Autodesk Inventor part; units mm, degrees
ref_plane "MSC_PT1" through (0, 0, 1.8) normal (0, 0, 1) x (1, 0, 0)
ref_plane "MSC_PT2" through (0, 0, 0) normal (0, 0, -1) x (-1, 0, 0)
ref_plane "MSC_PF1" through (0, 0, 0) normal (1, 0, 0) x (0, 1, 0)
sketch "Sketch1" plane through (0, 0, 0) normal (0, 0, 1) x (1, 0, 0)
  circle A0 centre (0, 0) radius 2.75 construction
  line L0 (-2.75, 1.5877) -> (-2.75, -1.5877)
  line L1 (-2.75, -1.5877) -> (0, -3.1754)
  line L2 (0, -3.1754) -> (2.75, -1.5877)
  line L3 (2.75, -1.5877) -> (2.75, 1.5877)
  line L4 (2.75, 1.5877) -> (0, 3.1754)
  line L5 (0, 3.1754) -> (-2.75, 1.5877)
  line L6 (0, 4.4456) -> (0, -4.4456)
  line L7 (-3.85, 0) -> (3.85, 0)
  point P0 (0, 0)
  dimension "ParS" = 5.5
extrude "Extrusion1" add sketch "Sketch1" along normal blind 1.8
sketch "Sketch2" plane through (0, 0, 1.8) normal (0, 0, 1) x (1, 0, 0)
  point P0 (0, 0)
  point P1 (0, 0)
hole "Hole1" at (0, 0, 1.8) direction (0, 0, -1) diameter 2.459 end through all
ref_plane "MSC_PT1" through (0, 0, 1.8) normal (0, 0, 1) x (1, 0, 0)
ref_plane "MSC_PT2" through (0, 0, 0) normal (0, 0, -1) x (-1, 0, 0)
ref_plane "MSC_PF1" through (0, 0, 0) normal (1, 0, 0) x (0, 1, 0)
chamfer "Chamfer1" distance 0.3 angle 45 2 edges at (0, 1.2295, 1.8) (0, 1.2295, 0)
equation "\"d17\" = 0.6 * PTC"
equation "\"d18\" = 0.6 * PTC"
equation "\"d4\" = M"
equation "\"PTC\" = 0.5"
equation "\"NND\" = 3"
equation "\"THREADDIA\" = NND"
properties part number "ISO 4036 - M3" material "Steel, Mild"
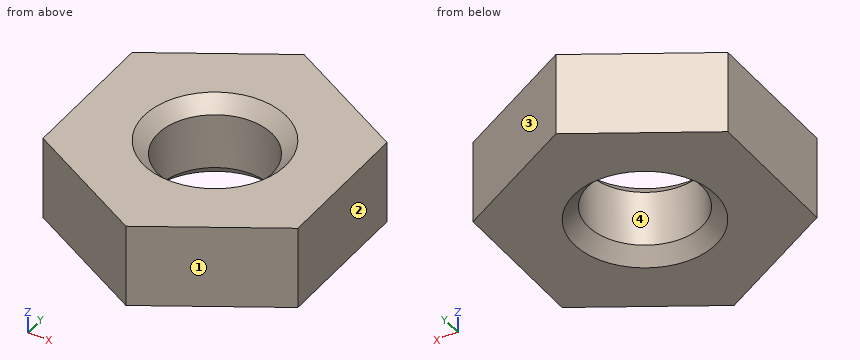
The listing builds one solid part. Answer for the finished solid, in the listing's coordinates (mm). Face numbers are marked on the shaded views. Round coordinates to 2 decimals unless told otherwise and drop trailing zeros. Loops run counter-clockwise (first coordinate to the right, second up) from the corner with the lowest first, then second, coordinate; pieces in that order, holes last. Notation, with made-up numbers: M 20.25,38 L 39.25,38 A12 ccw 39.25,61 Z; hole C 38,38.5 d1. An arc over 180 degrees is marked long. Write each question's results on one line, items separated by ' | '. Start each with the question number.
1) Find section D-D on y = -2. Write down the section's boundary in (x, z), plus the area to 3 significant figures.
2) Determine the mould class of the marked faces 1, 2, 3 and 4 for opening direction Y: pulls with the +Y half, pulls with the -Y half, needs draft (parallel to the pull), parting line crosses it, or undercut.
3) Find section C-C on z = 0.2. Write down the section's boundary in (x, y), plus the area to 3 significant figures.
4) Straight lines are drawn through the part: probe 1 along X at (y, z) = (0, 0.7); probe 2 along Y at (x, z) = (0.9, 1.05); probe 3 along X at (y, z) = (-0.5, 1.15). For each, find the intervals that lie inside material, in ascending order.
5) Find section B-B on y = 0. Write down the section's boundary in (x, z).
6) Each of these flat-tipped pins is pushed along its axis until it touches: pin 1 (1 mm diameter, centred on x = 1, z = 1, fed in from -Y); pin 2 (3 mm diameter, centred on x = 0, y = 0, fed in from +Z); pin 3 (1 mm diameter, centred on x = 1.5, z = 0.5, fed in from -Y). Where does it stop, or does it pass through?
7) Find section A-A on z = 0.75. Write down the section's boundary in (x, y), plus the area to 3 significant figures.
Final values:
1) outline: M -2.04,0 L 2.04,0 L 2.04,1.8 L -2.04,1.8 Z | area: 7.33 mm²
2) face 1: pulls with the -Y half | face 2: needs draft | face 3: pulls with the +Y half | face 4: undercut
3) outline: M -2.75,-1.59 L 0,-3.18 L 2.75,-1.59 L 2.75,1.59 L 0,3.18 L -2.75,1.59 Z; hole C 0,0 d2.66 | area: 20.6 mm²
4) probe 1: -2.75 to -1.23, 1.23 to 2.75 | probe 2: -2.66 to -0.84, 0.84 to 2.66 | probe 3: -2.75 to -1.12, 1.12 to 2.75
5) outline: M -2.75,0 L -1.53,0 L -1.23,0.3 L -1.23,1.5 L -1.53,1.8 L -2.75,1.8 Z; M 1.23,0.3 L 1.53,0 L 2.75,0 L 2.75,1.8 L 1.53,1.8 L 1.23,1.5 Z
6) pin 1: y = -2.89 | pin 2: z = 1.77 | pin 3: y = -2.6
7) outline: M -2.75,-1.59 L 0,-3.18 L 2.75,-1.59 L 2.75,1.59 L 0,3.18 L -2.75,1.59 Z; hole C 0,0 d2.46 | area: 21.4 mm²
